Model file for the job. Use its own axes, mm. A direction names the side the tool comes from. Give positions to 0.01 mm unless a question says otherwise; leave off trailing zeros. Order: outer loops, then holes, each group sorted by start corner. A loop starts at its lowest first (then second) coordinate and runs counter-clockwise, first axis right, second up. Notation, with made-up numbers: M -6,71 L 17,71 A25 ccw 17,88 Z; hole C -26.5,86.25 d8. An arc over 180 degrees is marked long. Return JSON: item names as keys, results as strings. Group by question number.
1. Wall check: probe 1 along Y at (x, z) = (38, -1.45); probe 2 along Y at (x, z) = (18, -2.75); probe 3 along X at (y, z) = (99, -0.2). Give the ranges that are in metal, low to high. Write a range as [from, to].
2. 3-axis set-ups, long thin cutter, end or side, ignore diameter. For faces 1 (the face through (2, 24.286, -2)), 2 (the face through (2, 121.429, -2)), 3 (the face through (20, 166, -2)), 4 (the face through (36, 156, -2)), 5 (the face through (24, 2, -2)): which of +Z, -Z, +X, -X, +Y, -Y reach the whole face in a straight line?
3. Slice it at A-A on y = 106. List the corners of the cut face in (x, z).
4. Pin check, flat tips, straight feed: pin 1 (1.2 mm diameter, centred on x = 38, z = -2.5, fed in from +Y); pin 2 (1 mm diameter, centred on y = 103, z = -3.5, fed in from +X); pin 3 (2 mm diameter, centred on y = 1, z = -1, fed in from -X); pin 4 (2 mm diameter, centred on x = 25.5, y = 66, fed in from +Z). Stop position of each tip, or through.
from build123d import *

# Parameters (mm, degrees)
BUITENAFMETING_RECHTHOEK_W  = 40
BUITENAFMETING_RECHTHOEK_H  = 170
PLAAT_DEPTH                 = 4
TAND_HOR_W                  = 8
TAND_HOR_H                  = 4
TAND_BOVEN_DEPTH            = 5
TANDEN_PATROON_BOVEN_COUNT  = 3
TANDEN_PATROON_BOVEN_PITCH  = 16
TAND_VER_W                  = 4
TAND_VER_H                  = 24.285714286
TAND_LINKS_DEPTH            = 5
TANDEN_PATROON_LINKS_COUNT  = 4
TANDEN_PATROON_LINKS_PITCH  = 48.571428571
TAND_O_W                    = 8
TAND_O_H                    = 4
TAND_ONDER_DEPTH            = 5
TANDEN_PATROON_ONDER_COUNT  = 3
TANDEN_PATROON_ONDER_PITCH  = 16
TAND_R_W                    = 4
TAND_R_H                    = 24.285714286
TAND_RECHTS_DEPTH           = 5
TANDEN_PATROON_RECHTS_COUNT = 4
TANDEN_PATROON_RECHTS_PITCH = 48.571428571


with BuildPart() as part:
    # Buitenafmeting Rechthoek → Plaat (new body)
    with BuildSketch(Plane.XY):
        with Locations((20, 85)):
            Rectangle(BUITENAFMETING_RECHTHOEK_W, BUITENAFMETING_RECHTHOEK_H)
    extrude(amount=-PLAAT_DEPTH)

    # Tand Hor → Tand Boven (cut, through all)
    with BuildSketch(Plane.XY):
        with Locations((4, 168)):
            Rectangle(TAND_HOR_W, TAND_HOR_H)
    tand_boven = extrude(amount=-TAND_BOVEN_DEPTH, mode=Mode.SUBTRACT)

    # Tanden Patroon Boven: Tand Boven ×3
    with Locations(*[(i * TANDEN_PATROON_BOVEN_PITCH, 0, 0) for i in range(1, TANDEN_PATROON_BOVEN_COUNT)]):
        add(tand_boven, mode=Mode.SUBTRACT)

    # Tand Ver → Tand Links (cut, through all)
    with BuildSketch(Plane.XY):
        with Locations((2, 157.857142857)):
            Rectangle(TAND_VER_W, TAND_VER_H)
    tand_links = extrude(amount=-TAND_LINKS_DEPTH, mode=Mode.SUBTRACT)

    # Tanden Patroon Links: Tand Links ×4
    with Locations(*[(0, -i * TANDEN_PATROON_LINKS_PITCH, 0) for i in range(1, TANDEN_PATROON_LINKS_COUNT)]):
        add(tand_links, mode=Mode.SUBTRACT)

    # Tand O → Tand Onder (cut, through all)
    with BuildSketch(Plane.XY):
        with Locations((4, 2)):
            Rectangle(TAND_O_W, TAND_O_H)
    tand_onder = extrude(amount=-TAND_ONDER_DEPTH, mode=Mode.SUBTRACT)

    # Tanden Patroon Onder: Tand Onder ×3
    with Locations(*[(i * TANDEN_PATROON_ONDER_PITCH, 0, 0) for i in range(1, TANDEN_PATROON_ONDER_COUNT)]):
        add(tand_onder, mode=Mode.SUBTRACT)

    # Tand R → Tand Rechts (cut, through all)
    with BuildSketch(Plane.XY):
        with Locations((38, 157.857142857)):
            Rectangle(TAND_R_W, TAND_R_H)
    tand_rechts = extrude(amount=-TAND_RECHTS_DEPTH, mode=Mode.SUBTRACT)

    # Tanden Patroon Rechts: Tand Rechts ×4
    with Locations(*[(0, -i * TANDEN_PATROON_RECHTS_PITCH, 0) for i in range(1, TANDEN_PATROON_RECHTS_COUNT)]):
        add(tand_rechts, mode=Mode.SUBTRACT)


solid = part.part
Result:
{
 "1": {"probe 1": "y = [24.29, 48.57], [72.86, 97.14], [121.43, 145.71]", "probe 2": "y = [4, 166]", "probe 3": "x = [4, 36]"},
 "2": {"face 1": "+Z, -Z, -X, -Y", "face 2": "+Z, -Z, -X", "face 3": "+Z, -Z, +Y", "face 4": "+Z, -Z, +X, +Y", "face 5": "+Z, -Z, -Y"},
 "3": {"outline": "M 4,-4 L 36,-4 L 36,0 L 4,0 Z"},
 "4": {"pin 1": "stops at y = 145.71", "pin 2": "stops at x = 36", "pin 3": "stops at x = 8", "pin 4": "stops at z = 0"}
}
